from build123d import *

# Parameters (mm, degrees)
SKETCH1_W           = 15.875
SKETCH1_H           = 12.7
BOSS_EXTRUDE1_DEPTH = 2.54
FILLET1_R           = 0.635
SHELL1_START        = 0.635
SHELL1_OUTLINE_W    = 1.905
SHELL1_OUTLINE_H    = 11.43
SHELL1_DEPTH        = 14.605
SKETCH2_R           = 2.54
BOSS_EXTRUDE2_DEPTH = 1.905


# Read off the part's stored shape, not the designer's step: Shell1
with BuildPart() as part:
    # Sketch1 → Boss-Extrude1 (new body)
    with BuildSketch(Plane(origin=(0, 0, 0), x_dir=(1, 0, 0), z_dir=(0, 1, 0))):
        with Locations((7.9375, 6.35)):
            Rectangle(SKETCH1_W, SKETCH1_H)
    extrude(amount=BOSS_EXTRUDE1_DEPTH)

    # Fillet1
    fillet1_edges = [part.edges().sort_by_distance(p)[0] for p in [
        (0, 1.27, -12.7),
        (15.875, 1.27, -12.7),
        (15.875, 1.27, 0),
        (0, 1.27, 0),
    ]]
    fillet(fillet1_edges, radius=FILLET1_R)

    # Shell1 outline → Shell1 (cut)
    with BuildSketch(Plane.YZ.offset(SHELL1_START)):
        with Locations((0.9525, -6.35)):
            Rectangle(SHELL1_OUTLINE_W, SHELL1_OUTLINE_H)
    extrude(amount=SHELL1_DEPTH, mode=Mode.SUBTRACT)

    # Sketch2 → Boss-Extrude2 (add)
    with BuildSketch(Plane(origin=(0, 1.905, 0), x_dir=(-1, 0, 0), z_dir=(0, -1, 0))):
        with Locations(Location((-7.9375, 6.35, 0), (0, 0, 270))):
            Circle(SKETCH2_R)
    extrude(amount=BOSS_EXTRUDE2_DEPTH)


solid = part.part
Design review of the part built by this model. Coordinates are the model's own, in mm. A direction names the side the tool comes from. Coordinates: 2 decimals unless noted, no trailing zeros. Loops run counter-clockwise (first coordinate to the right, second up) from the corner with the lowest first, then second, coordinate; pieces in that order, holes last. Notation, with made-up numbers: (41, 25) -> (97, 25) arc R23 cw to (97, 54) -> close; hole circle Ø11 at (80.25, 25). An arc over 180 degrees is marked (long way). Use a Markdown table: item, result. Add a question column.
Item 1: The part is to be moulded in two halves that separate along Z. For faces 1 (the flat face through (8, 1, 0)), 2 (the flat face through (15.24, 1, -6)), 3 (the flat face through (8, 1, -0.635)), 4 (the flat face through (8, 0, -6)), say which applies: +Z half, -Z half, draft (parallel to the pull), parting line (faces both ways), or undercut.
Item 2: We need section C-C, the plane z = -10. Write out the cut boundary in (x, y) (3 decimals), and give its area (3 significant figures).
Item 3: Wall thickness on L1, parallel to X at y = 0.95, z = -9 (3 decimals); L2, parallel to Z at x = 14, y = 1.05 (3 decimals); L3, parallel to Z at x = 9.5, y = 0.55 (3 decimals): over which ranges is each line inside the solid? List them lowest first. Write a range as from..to.
Item 4: We need section B-B, the plane x = 11. Write out the cut boundary in (y, z) (3 decimals).
Item 5: We need section A-A, the plane y = 1. Count the separate pieces of the cut face and the enclosed holes in it, and give its area (3 significant figures).
Item 6: Machinability: for faces 5 (the flat face through (7.3, 0, -0.3)), 6 (the flat face through (8, 1, -12.065)), which of the approach directions +Z, -Z, +X, -X, +Y, -Y give a long, thin tool a straight path to every point of the face, cutting with its end or side? Answer none if there is none.
Item 7: We need section D-D, the plane z = -6.35. Write out the cut boundary in (x, y) (1 decimal), and give its area (3 significant figures).
Numbers:
| question | item | result |
|---|---|---|
| 1 | face 1 | +Z half |
| 1 | face 2 | undercut |
| 1 | face 3 | undercut |
| 1 | face 4 | draft |
| 2 | outline | (0, 0) -> (0.635, 0) -> (0.635, 1.905) -> (15.24, 1.905) -> (15.24, 0) -> (15.875, 0) -> (15.875, 2.54) -> (0, 2.54) -> close |
| 2 | area | 12.5 mm^2 |
| 3 | L1 | x = 0..0.635, 15.24..15.875 |
| 3 | L2 | z = -12.7..-12.065, -0.635..0 |
| 3 | L3 | z = -12.7..-12.065, -8.353..-4.347, -0.635..0 |
| 4 | outline | (0, -12.7) -> (2.54, -12.7) -> (2.54, 0) -> (0, 0) -> (0, -0.635) -> (1.905, -0.635) -> (1.905, -12.065) -> (0, -12.065) -> close |
| 5 | separate pieces | 2 |
| 5 | enclosed holes | 1 |
| 5 | area | 54.6 mm^2 |
| 6 | face 5 | +Z, -Z, +X, -X, -Y |
| 6 | face 6 | -Y |
| 7 | outline | (0, 0) -> (0.6, 0) -> (0.6, 1.9) -> (5.4, 1.9) -> (5.4, 0) -> (10.5, 0) -> (10.5, 1.9) -> (15.2, 1.9) -> (15.2, 0) -> (15.9, 0) -> (15.9, 2.5) -> (0, 2.5) -> close |
| 7 | area | 22.2 mm^2 |
